Verification items for the finished model (mm, model axes). Face numbers are marked on the shaded views. A direction names the side the tool comes from. Give positions to 0.01 mm unless a question says otherwise; leave off trailing zeros. Write each loop counter-clockwise with the first axis right and the second up, starting at its lowest first coordinate (ties: lowest second). Pieces come first, ordered by that corner, then holes.
from build123d import *

# Parameters (mm, degrees)
F2_W     = 64
F2_H     = 64
F2_W_2   = 62
F2_H_2   = 62
F3_DEPTH = 17
F4_DEPTH = 1
F5_R     = 4


with BuildPart() as f3:
    # F2 (on Top) → F3 (new body)
    with BuildSketch(Plane.XY):
        with Locations((31, -31)):
            Rectangle(F2_W, F2_H)
        with Locations((31, -31)):
            Rectangle(F2_W_2, F2_H_2, mode=Mode.SUBTRACT)
    extrude(amount=F3_DEPTH)

    # F2 (on Top) → F4 (join)
    with BuildSketch(Plane.XY):
        with Locations((31, -31)):
            Rectangle(F2_W, F2_H)
        with Locations((31, -31)):
            Rectangle(F2_W_2, F2_H_2, mode=Mode.SUBTRACT)
        with Locations((31, -31)):
            Rectangle(F2_W_2, F2_H_2)
    extrude(amount=-F4_DEPTH)

    # F5
    f5_edges = [f3.edges().sort_by_distance(p)[0] for p in [
        (0, -31, 0),
        (31, 0, 0),
        (62, -31, 0),
        (31, -62, 0),
        (31, 1, -1),
        (-1, -31, -1),
        (31, -63, -1),
        (63, -31, -1),
        (0, -62, 8.5),
        (0, 0, 8.5),
        (62, 0, 8.5),
        (62, -62, 8.5),
        (-1, 1, 8),
        (63, 1, 8),
        (63, -63, 8),
        (-1, -63, 8),
    ]]
    fillet(f5_edges, radius=F5_R)


solid = f3.part
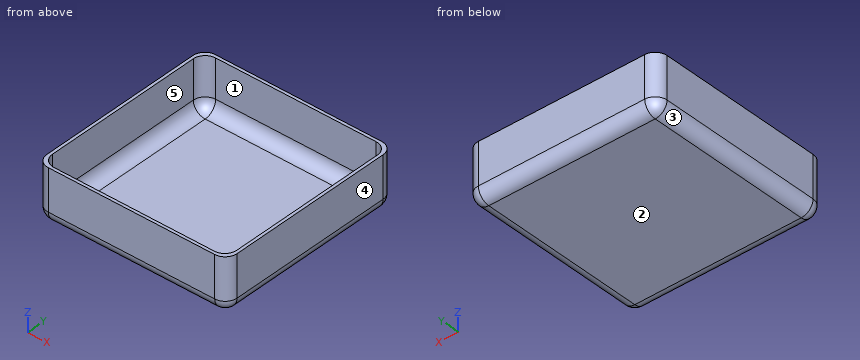
Item 1: Sectioned sample at C-C on y = -5. Record the cut outline in (x, z), then the cut area to 3 significant figures.
Answer key:
outline: (-1, 3) arc R4 ccw to (3, -1) - (59, -1) arc R4 ccw to (63, 3) - (63, 17) - (62, 17) - (62, 4) arc R4 cw to (58, 0) - (4, 0) arc R4 cw to (0, 4) - (0, 17) - (-1, 17) - close
area: 98.0 mm2
Item 2: Sectioned sample at B-B on x = 31. Record the cut outline in (y, z).
Answer key:
outline: (-63, 3) arc R4 ccw to (-59, -1) - (-3, -1) arc R4 ccw to (1, 3) - (1, 17) - (0, 17) - (0, 4) arc R4 cw to (-4, 0) - (-58, 0) arc R4 cw to (-62, 4) - (-62, 17) - (-63, 17) - close
Item 3: Sectioned sample at A-A on z = 9. Record the cut outline in (x, y), then the cut area to 3 significant figures.
Answer key:
outline: (-1, -59) arc R4 ccw to (3, -63) - (59, -63) arc R4 ccw to (63, -59) - (63, -3) arc R4 ccw to (59, 1) - (3, 1) arc R4 ccw to (-1, -3) - close; hole (0, -58) arc R4 ccw to (4, -62) - (58, -62) arc R4 ccw to (62, -58) - (62, -4) arc R4 ccw to (58, 0) - (4, 0) arc R4 ccw to (0, -4) - close
area: 252 mm2
Item 4: Scan lines: line 1 along X through (y, z) = (-54.5, 14); line 2 along Y through (x, z) = (14, 11.5); line 3 along Z through (x, y) = (7, -41.5). Record each from-to range of solid material in increasing order.
Answer key:
line 1: x = -1 to 0, 62 to 63
line 2: y = -63 to -62, 0 to 1
line 3: z = -1 to 0
Item 5: Sectioned sample at D-D on z = 1.75. Record the cut outline in (x, y), then the cut area to 3 significant figures.
Answer key:
outline: (-0.8, -59) arc R3.8 ccw to (3, -62.8) - (59, -62.8) arc R3.8 ccw to (62.8, -59) - (62.8, -3) arc R3.8 ccw to (59, 0.8) - (3, 0.8) arc R3.8 ccw to (-0.8, -3) - close; hole (0.69, -58) arc R3.31 ccw to (4, -61.31) - (58, -61.31) arc R3.31 ccw to (61.31, -58) - (61.31, -4) arc R3.31 ccw to (58, -0.69) - (4, -0.69) arc R3.31 ccw to (0.69, -4) - close
area: 368 mm2
Item 6: Release check for a two-part mould opening along X. For the marked faces 1, 2 and 3 record: released by +X, released by -X, zero draft, split by the parting line, or undercut.
Answer key:
face 1: undercut
face 2: zero draft
face 3: released by -X
Item 7: Set-up check for the marked faces 4 and 5: record each of +Z, -Z, +X, -X, +Y, -Y from which the full face is reachable in a straight line by a thin tool's end or side.
Answer key:
face 4: +Z, -Z, +X, +Y, -Y
face 5: +Z
Item 8: Depth check by flat-ended pin: pin 1 (1 mm diameter, centred on x = 28, y = -44.5, fed in from +Z). Enter the tip coordinate at first touch or a pass-through.
Answer key:
pin 1: stops at z = 0
